Part print with two shaded views. Sizes in mm from the minimum x, y, z corner. Give positions to 0.01 mm unless a question says otherwise; leave off trailing zeros. Order: outer loops, then holes, each group sorted by start corner. A loop starts at its lowest first (then second) coordinate and runs counter-clockwise, first axis right, second up. Notation, with made-up numbers: M 44.25,12.25 L 61.25,12.25 A20 ccw 61.25,28.25 Z; hole C 76.5,-4 d4. An arc over 180 degrees is marked long. Return JSON: item names as keys, results as strings. Group by question number.
1. Slice it at A-A on z = 2.75. List the corners of the cut face in (x, y) (3 decimals), then the cut area to 3 significant figures.
2. Pin check, flat tips, straight feed: pin 1 (8 mm diameter, centred on y = 21, z = 6, fed in from +X); pin 2 (8 mm diameter, centred on x = 1396, z = 5, fed in from -Y). Stop position of each tip, or through.
3. Wall check: probe 1 along X at (y, z) = (23.5, 4). Give the ranges that are in metal, low to high. Write a range as [from, to].
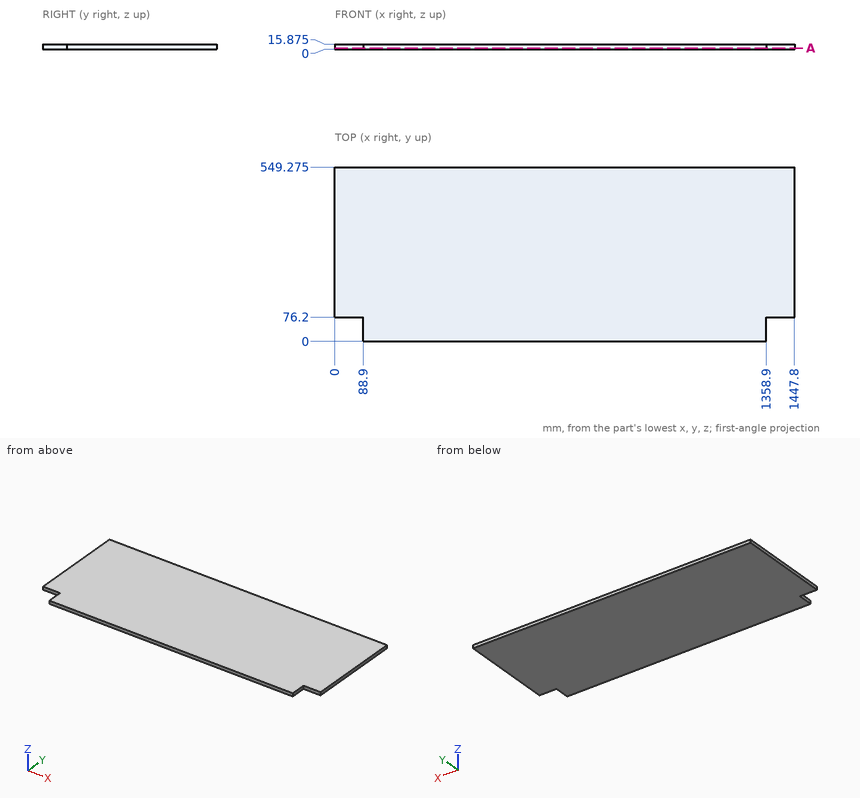
Result:
{
 "1": {"outline": "M 0,76.2 L 88.9,76.2 L 88.9,0 L 1358.9,0 L 1358.9,76.2 L 1447.8,76.2 L 1447.8,549.275 L 0,549.275 Z", "area": "782,000 mm2"},
 "2": {"pin 1": "stops at x = 1358.9", "pin 2": "stops at y = 76.2"},
 "3": {"probe 1": "x = [88.9, 1358.9]"}
}
